Source: CAD feature listing. Evaluate the final solid. Frame: model axes, mm. Round coordinates to 2 decimals unless told otherwise and drop trailing zeros. Write each loop counter-clockwise with the first axis right and the second up, starting at its lowest first coordinate (ties: lowest second). Pieces come first, ordered by that corner, then holes. Notation, with made-up numbers: M 58,11 L 69,11 A36 cw 69,47 Z; hole C -5,-8.75 d3. An arc over 180 degrees is marked long. Use a Markdown table: item, result.
Autodesk Inventor part; units mm, degrees
ref_plane "Work Plane1" through (0, 0, 0) normal (0, -1, 0) x (1, 0, 0)
ref_plane "YZ Plane" through (0, 0, 0) normal (1, 0, 0) x (0, 1, 0)
ref_plane "XZ Plane" through (0, 0, 0) normal (0, 1, 0) x (-1, 0, 0)
sketch "草图1" plane through (0, 0, 0) normal (1, 0, 0) x (0, 1, 0)
  circle A0 centre (0, 0) radius 7.7
  circle A1 centre (0, 0) radius 5.1
  dimension "d0" = 10.2
  dimension "d1" = 15.4
extrude "轴承体" add sketch "草图1" along normal blind 2.6
sketch "草图2" plane through (0, 0, 0) normal (0, 0, 1) x (1, 0, 0)
  line L0 (0, -5.1) -> (0, 5.1)
  line L1 (2.6, 7.7) -> (2.6, -7.7)
  line L2 (-1.2, 0) -> (7.2, 0)
  line L3 (0, -0.52) -> (2.6, 0.3248)
  line L4 (0, 0.52) -> (2.6, 1.3648)
  dimension "d4" = 0.52
  dimension "d5" = 0.52
  dimension "d6" = 72
extrude "切口" cut sketch "草图2" along normal up to next contours L0 L2 L3 | L0 L4 L1 L3 L2
ref_plane "Work Plane1" through (0, 0, 0) normal (0, -1, 0) x (1, 0, 0)
equation "\"d0\" = SD1"
equation "\"d1\" = SD2"
equation "\"d2\" = SD"
equation "\"d4\" = 0.2 * SD"
equation "\"d5\" = 0.2 * SD"
equation "\"d6\" = FAWI"
equation "\"d7\" = SD"
equation "\"SD1\" = 10.2"
equation "\"SD2\" = 15.4"
equation "\"SD\" = 2.6"
equation "\"FAWI\" = 72deg"
properties part number "垫圈 GB 93-87 10" material "钢，软"
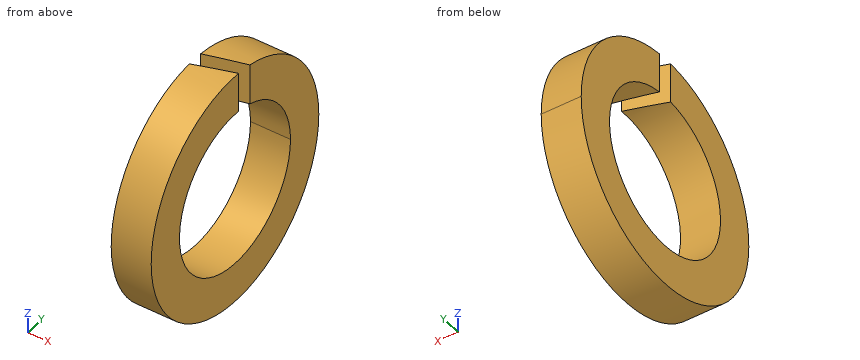
Q1. Line query: L1, parallel to Z at x = 2, y = 0; L2, parallel to Z at x = 2.4, y = 2.5. Output: solid intervals per line, ascending.
Results are:
| item | result |
|---|---|
| L1 | -7.7 to -5.1, 5.1 to 7.7 |
| L2 | -7.28 to -4.45, 4.45 to 7.28 |
Q2. Section A-A on z = -1.5. Return loops of the section in (x, y).
Results are:
| item | result |
|---|---|
| outline | M 0,-7.55 L 2.6,-7.55 L 2.6,-4.87 L 0,-4.87 Z; M 0,4.87 L 2.6,4.87 L 2.6,7.55 L 0,7.55 Z |
Q3. Section D-D on y = 6.5. Return loops of the section in (x, z), plus the area to 3 significant figures.
Results are:
| item | result |
|---|---|
| outline | M 0,-4.13 L 2.6,-4.13 L 2.6,4.13 L 0,4.13 Z |
| area | 21.5 mm^2 |
Q4. Section C-C on x = 2.2. Return loops of the section in (y, z), plus the area to 3 significant figures.
Results are:
| item | result |
|---|---|
| outline | M 0.19,5.1 L 0.19,7.7 A7.7 ccw long 1.23,7.6 L 1.23,4.95 A5.1 cw long Z |
| area | 102 mm^2 |
Q5. First-contact query: pin 1 Ø9 at (y, z) = (0, 0) entering from +X. Flat tip, straight axial feed; report the tip coordinate or a pass-through.
Results are:
| item | result |
|---|---|
| pin 1 | through |
Q6. Section B-B on y = 1.75. Return loops of the section in (x, z), plus the area to 3 significant figures.
Results are:
| item | result |
|---|---|
| outline | M 0,-7.5 L 2.6,-7.5 L 2.6,-4.79 L 0,-4.79 Z; M 0,4.79 L 2.6,4.79 L 2.6,7.5 L 0,7.5 Z |
| area | 14.1 mm^2 |
